Part print with two shaded views. Sizes in mm from the minimum x, y, z corner. A direction names the side the tool comes from. Coordinates: 2 decimals unless noted, no trailing zeros. Loops run counter-clockwise (first coordinate to the right, second up) from the corner with the lowest first, then second, coordinate; pieces in that order, holes last.
Item 1: Drill centre line: line 1 along X through (y, z) = (5.5, 74.5). Where is it in solid material? Low to high.
Item 2: Cut at A-A (y = 17). List the corners of the cut face in (x, z), and give its area (3 significant figures).
Item 3: Mould opens along X. For the marked faces 3, 4 and 5 say: released by +X, released by -X, zero draft, split by the parting line, or undercut.
Item 4: Cut at C-C (z = 18). List the corners of the cut face in (x, y).
Item 5: 3-axis set-ups, long thin cutter, end or side, ignore diameter. For the marked faces 1 and 2: which of +Z, -Z, +X, -X, +Y, -Y reach the whole face in a straight line?
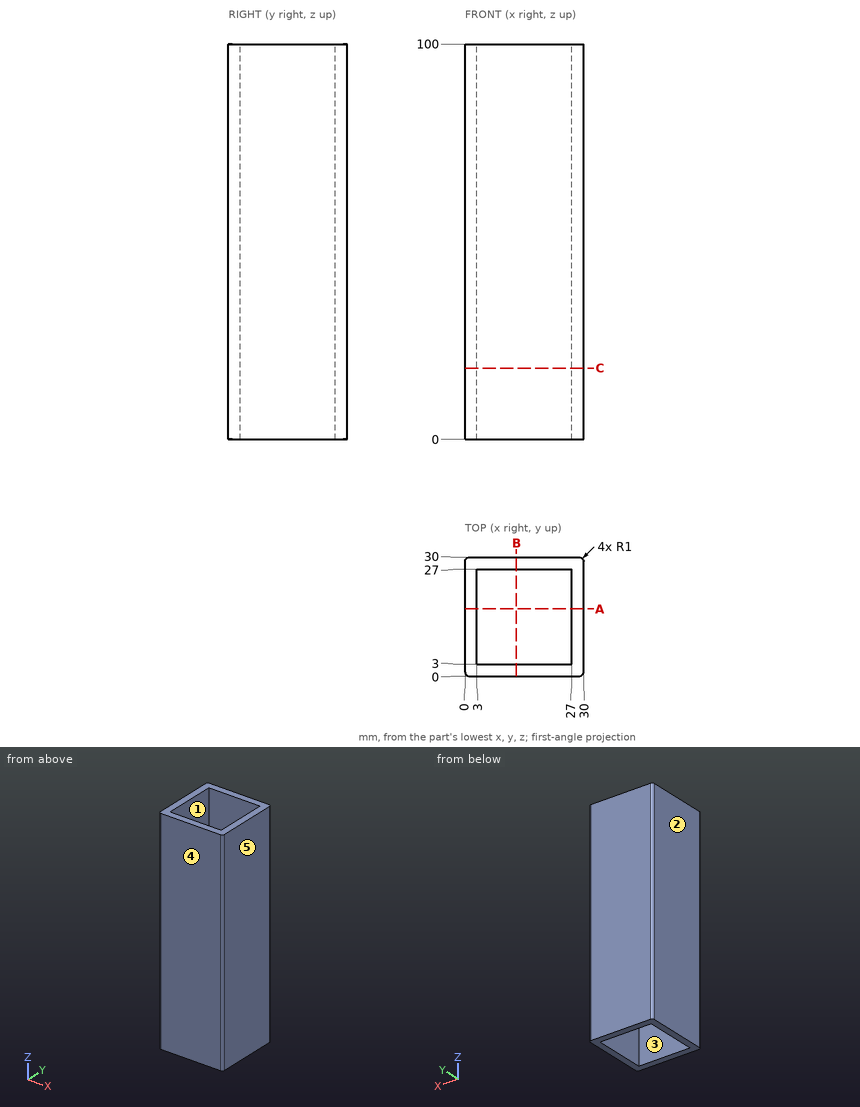
Filled sheet:
1. line 1: x = 0 to 3, 27 to 30
2. outline: (0, 0) - (3, 0) - (3, 100) - (0, 100) - close; (27, 0) - (30, 0) - (30, 100) - (27, 100) - close
2. area: 600 mm2
3. face 3: undercut
3. face 4: zero draft
3. face 5: released by +X
4. outline: (0, 1) arc R1 ccw to (1, 0) - (29, 0) arc R1 ccw to (30, 1) - (30, 29) arc R1 ccw to (29, 30) - (1, 30) arc R1 ccw to (0, 29) - close; hole (3, 3) - (27, 3) - (27, 27) - (3, 27) - close
5. face 1: +Z, -Z
5. face 2: +Z, -Z, -X, +Y, -Y
